from build123d import *

# Parameters (mm, degrees)
F0_W      = 33
F0_H      = 14
F1_DEPTH  = 10
F2_W      = 15
F2_H      = 14
F3_DEPTH  = 12
F4_R      = 7
F5_R      = 6.99999
F7_DEPTH  = 24.001
F8_W      = 18
F8_H      = 14
F9_DEPTH  = 15
F11_DEPTH = 25
F13_R     = 6.99999
F12_W     = 3.3
F12_H     = 15
F14_DEPTH = 25
F15_R     = 2.5
F16_DEPTH = 3.6


# Not quite as in the source:
# - a fillet or chamfer is up to 0.001 mm smaller than in the source, because OpenCascade refuses the exact size


with BuildPart() as f1:
    # F0 (on Top) → F1 (new body)
    with BuildSketch(Plane.XY):
        with Locations((16.5, -7)):
            Rectangle(F0_W, F0_H)
    extrude(amount=F1_DEPTH)

    # F2 (on face) → F3 (join)
    with BuildSketch(Plane(origin=(0, 0, 0), x_dir=(1, 0, 0), z_dir=(0, 0, -1))):
        with Locations((16.5, 7)):
            Rectangle(F2_W, F2_H)
    extrude(amount=F3_DEPTH)

    # F4
    f4_edges = [f1.edges().sort_by_distance(p)[0] for p in [
        (16.5, 0, -12),
    ]]
    fillet(f4_edges, radius=F4_R)

    # F5 (radius 7 in the source; OpenCascade refuses exactly that, so slightly less here)
    f5_edges = [f1.edges().sort_by_distance(p)[0] for p in [
        (16.5, -14, -12),
    ]]
    fillet(f5_edges, radius=F5_R)

    # F6 (on face) → F7 (cut, through all)
    with BuildSketch(Plane.YZ.offset(24)):
        with BuildLine():
            Line((-7, -10), (-7, -6))
            ThreePointArc((-7, -6), (-9, -8), (-7, -10))
        make_face()
        with BuildLine():
            ThreePointArc((-7, -10), (-5.5857864376, -9.4142135624), (-5, -8))
            ThreePointArc((-5, -8), (-5.5857864376, -6.5857864376), (-7, -6))
            Line((-7, -6), (-7, -10))
        make_face()
    extrude(amount=-F7_DEPTH, mode=Mode.SUBTRACT)

    # F8 (on face) → F9 (join)
    with BuildSketch(Plane.XY.offset(10)):
        with Locations((16.5, -7)):
            Rectangle(F8_W, F8_H)
    extrude(amount=F9_DEPTH)

    # F10 (on face) → F11 (cut)
    with BuildSketch(Plane(origin=(7.5, 0, 0), x_dir=(0, -1, 0), z_dir=(-1, 0, 0))):
        with BuildLine():
            Line((7, 22.4445006251), (7, 17.4445006251))
            ThreePointArc((7, 17.4445006251), (8.767766953, 18.1767336722), (9.5, 19.9445006251))
            ThreePointArc((9.5, 19.9445006251), (8.767766953, 21.7122675781), (7, 22.4445006251))
        make_face()
        with BuildLine():
            ThreePointArc((7, 22.4445006251), (4.5, 19.9445006251), (7, 17.4445006251))
            Line((7, 17.4445006251), (7, 22.4445006251))
        make_face()
    extrude(amount=-F11_DEPTH, mode=Mode.SUBTRACT)

    # F13 (radius 7 in the source; OpenCascade refuses exactly that, so slightly less here)
    f13_edges = [f1.edges().sort_by_distance(p)[0] for p in [
        (16.5, -14, 25),
        (16.5, 0, 25),
    ]]
    fillet(f13_edges, radius=F13_R)

    # F12 (on face) → F14 (cut)
    with BuildSketch(Plane.XZ.offset(14)):
        with Locations((21.35, 17.5)):
            Rectangle(F12_W, F12_H)
        with Locations((15.15, 17.5)):
            Rectangle(F12_W, F12_H)
    extrude(amount=-F14_DEPTH, mode=Mode.SUBTRACT)

    # F15 (on face) → F16 (cut)
    with BuildSketch(Plane(origin=(7.5, 0, 0), x_dir=(0, -1, 0), z_dir=(-1, 0, 0))):
        Polygon((4.7483339502, 16.0445006251), (9.2516660498, 16.0445006251), (11.5033320997, 19.9445006251), (9.2516660498, 23.8445006251), (4.7483339502, 23.8445006251), (2.4966679003, 19.9445006251), align=None)
        with Locations((7, 19.9445006251)):
            Circle(F15_R, mode=Mode.SUBTRACT)
    extrude(amount=-F16_DEPTH, mode=Mode.SUBTRACT)


solid = f1.part
Geometry: final body of the model. Coordinates: model frame, mm. A direction names the side the tool comes from. Round coordinates to 2 decimals unless told otherwise and drop trailing zeros. Loops run counter-clockwise (first coordinate to the right, second up) from the corner with the lowest first, then second, coordinate; pieces in that order, holes last.
Q1. Section A-A on x = 10. State how many separate pieces and enclosed holes the cut face has, plus the area to 3 significant figures.
Q2. Material intervals for L1, parallel to X at y = -13, z = 12.5; L2, parallel to X at y = -8, z = 17.5; L3, parallel to Z at x = 23.5, y = -8.5, sorted ascending.
Q3. Section D-D on y = -1.25. Return loops of the section in (x, z), plus the area to 3 significant figures.
Q4. Access query for faces 1 (the flat face through (19.7, -7, 17)), 2 (the flat face through (28, -7, 0)), 3 (the flat face through (29, -7, 10)), 4 (the flat face through (9.27, -10.39, 21.87)). Directions: +Z, -Z, +X, -X, +Y, -Y. A direction counts if a zero-diameter tool reaches every point of the face in a straight line with its end or side. Return the directions, or none.
Q5. Pull-direction query (Z, two-part tool) for faces 5 (the flat face through (7.5, -7.1, 15.7)), 6 (the flat face through (9.275, -10.362, 17.967)), 7 (the cylindrical face through (18.3, -12, 22.9)); classes: released by +Z, released by -Z, zero draft, split by the parting line, or undercut.
Q6. Section B-B on z = -8.5. Return loops of the section in (x, y), plus the area to 3 significant figures.
Q7. Pin query (flat end, axial travel): P1, Ø2, axis at x = 30.5, y = -9.5, coming from the +Z side; P2, Ø7, axis at x = 5, y = -6.5, coming from the -Z side; P3, Ø6, axis at y = -6.5, z = -8, coming from the -X side. Return the tip coordinate at first contact, or that it passes through.
Evaluation:
1. separate pieces: 1
1. enclosed holes: 2
1. area: 411 mm2
2. L1: x = 7.5 to 13.5, 16.8 to 19.7, 23 to 25.5
2. L2: x = 11.1 to 13.5, 16.8 to 19.7, 23 to 25.5
2. L3: z = -11.84 to -9.32, -6.68 to 17.94, 21.94 to 24.84
3. outline: (0, 0) - (9, 0) - (9, -8.99) - (24, -8.99) - (24, 0) - (33, 0) - (33, 10) - (25.5, 10) - (25.5, 21.99) - (23, 21.99) - (23, 10) - (19.7, 10) - (19.7, 21.99) - (16.8, 21.99) - (16.8, 10) - (13.5, 10) - (13.5, 21.99) - (7.5, 21.99) - (7.5, 10) - (0, 10) - close
3. area: 602 mm2
4. face 1: +Z, +Y, -Y
4. face 2: -Z, +X, +Y, -Y
4. face 3: +Z, +X, +Y, -Y
4. face 4: -X
5. face 5: zero draft
5. face 6: undercut
5. face 7: released by +Z
6. outline: (9, -13.06) - (24, -13.06) - (24, -8.94) - (9, -8.94) - close; (9, -5.06) - (24, -5.06) - (24, -0.94) - (9, -0.94) - close
6. area: 124 mm2
7. P1: stops at z = 10
7. P2: stops at z = 0
7. P3: stops at x = 9
